Could you check a few things on this model? Use its own coordinates, in mm. A direction names the side the tool comes from. Coordinates: 2 decimals unless noted, no trailing zeros. Loops run counter-clockwise (first coordinate to the right, second up) from the corner with the lowest first, then second, coordinate; pieces in that order, holes last.
from build123d import *

# Parameters (mm, degrees)
BOTTOM_FILLET_R = 0.4


with BuildPart() as part:
    # Sketch2 → Main Body (revolve)
    with BuildSketch(Plane(origin=(0, 0, 0), x_dir=(1, 0, 0), z_dir=(0, 1, 0))):
        with BuildLine():
            Line((2.1, 0), (5.45, 0))
            ThreePointArc((5.45, 0), (5.101347861, -1.918006778), (4.1, -3.590612761))
            Line((4.1, -3.590612761), (4.1, -2.4))
            Line((4.1, -2.4), (1.25, -2.4))
            Line((1.25, -2.4), (1.25, -1.937095277))
            ThreePointArc((1.25, -1.937095277), (1.876107285, -1.16695398), (2.1, -0.2))
            Line((2.1, -0.2), (2.1, 0))
        make_face()
    revolve(axis=Axis((0, 0, 0), (0, 0, 1)))

    # Bottom Fillet
    bottom_fillet_edges = [part.edges().sort_by_distance(p)[0] for p in [
        (-5.45, 0, 0),
        (-2.1, 0, 0),
    ]]
    fillet(bottom_fillet_edges, radius=BOTTOM_FILLET_R)


solid = part.part
(1) For pin 1 (2 mm diameter, centred on x = -3.5, z = 1, fed in from -Y); pin 2 (1.5 mm diameter, centred on y = 1.5, z = 2.5, fed in from -X); pin 3 (3 mm diameter, centred on x = 0, y = 0, fed in from +Z), each with a flat end and sliding along its axis, tell me the tip position at first contact or that it passes through.
Answers:
pin 1: stops at y = -4.77
pin 2: stops at x = -5
pin 3: stops at z = 2.4
(2) We'd pull the mould along Y, two halves only. Please class faces 1 (the face through (-0.534, 4.065, 2.987)), 2 (the face through (0, 3, 0)): +Y half, -Y half, draft (parallel to the pull), parting line (faces both ways), or undercut.
Answers:
face 1: undercut
face 2: draft
(3) I need wall thicknesses on probe 1 along X at (y, z) = (0.75, 1.55); probe 2 along Z at (x, y) = (-1.5, -3.5); probe 3 along X at (y, z) = (0.5, 3.05). Which ranges of each line are inside material? Lowest first, please.
Answers:
probe 1: x = -5.17 to -1.46, 1.46 to 5.17
probe 2: z = 0 to 2.4
probe 3: x = -4.49 to -4.07, 4.07 to 4.49
(4) Which directions (+Z, -Z, +X, -X, +Y, -Y) give clear straight access to the entire face, cutting with the end or side of a thin tool? Please do faces 3 (the face through (-1, -1, 2.4)), 4 (the face through (-0.27, -1.22, 2.17)).
Answers:
face 3: +Z
face 4: +Z, -Z
(5) Imagine slicing it at A-A, the plane z = 2.2. Write out the boundary of the cut face in (x, y).
Answers:
outline: circle Ø9.97 at (0, 0); hole circle Ø2.5 at (0, 0)
